Geometry: final body of the model. Coordinates: model frame, mm. Give positions to 0.01 mm unless a question says otherwise; leave off trailing zeros. Write each loop counter-clockwise with the first axis right and the second up, starting at its lowest first coordinate (ties: lowest second). Pieces come first, ordered by that corner, then holes.
from build123d import *

# Parameters (mm, degrees)
SKETCH1_W          = 520
SKETCH1_H          = 430
BASE_FLANGE1_DEPTH = 4.78
SKETCH6_R          = 4.5
CUT_EXTRUDE1_DEPTH = 10
CHAMFER1_SIZE      = 80
SKETCH7_R          = 4.5
CUT_EXTRUDE2_DEPTH = 10
SKETCH8_R          = 4.25
CUT_EXTRUDE3_DEPTH = 10
SKETCH9_R          = 4.5
CUT_EXTRUDE4_DEPTH = 10
CUT_EXTRUDE5_DEPTH = 10
CHAMFER2_SIZE      = 3


# Sheet-metal steps are written as plain solids
with BuildPart() as part:
    # Sketch1 → Base-Flange1 (new body)
    with BuildSketch(Plane(origin=(0, 0, 0), x_dir=(1, 0, 0), z_dir=(0, 1, 0))):
        with Locations((0, -215)):
            Rectangle(SKETCH1_W, SKETCH1_H)
    extrude(amount=-BASE_FLANGE1_DEPTH)

    # Sketch6 → Cut-Extrude1 (cut)
    with BuildSketch(Plane(origin=(0, 0, 0), x_dir=(1, 0, 0), z_dir=(0, 1, 0))):
        with Locations(Location((62.5, -14.9625, 0), (0, 0, 270))):
            Circle(SKETCH6_R)
        with Locations(Location((0, -14.9625, 0), (0, 0, 270))):
            Circle(SKETCH6_R)
        with Locations(Location((-62.5, -14.9625, 0), (0, 0, 270))):
            Circle(SKETCH6_R)
    extrude(amount=-CUT_EXTRUDE1_DEPTH, mode=Mode.SUBTRACT)

    # Chamfer1
    chamfer1_edges = [part.edges().sort_by_distance(p)[0] for p in [
        (260, -2.39, 430),
        (-260, -2.39, 430),
    ]]
    chamfer(chamfer1_edges, length=CHAMFER1_SIZE)

    # Sketch7 → Cut-Extrude2 (cut)
    with BuildSketch(Plane(origin=(0, 0, 0), x_dir=(1, 0, 0), z_dir=(0, 1, 0))):
        with Locations(Location((-223.749160028, -139.138800169, 0), (0, 0, 270))):
            Circle(SKETCH7_R)
        with Locations(Location((-223.749160028, -274.331266718, 0), (0, 0, 270))):
            Circle(SKETCH7_R)
        with Locations(Location((223.749160028, -274.331266718, 0), (0, 0, 90))):
            Circle(SKETCH7_R)
        with Locations(Location((223.749160028, -139.138800169, 0), (0, 0, 90))):
            Circle(SKETCH7_R)
    extrude(amount=-CUT_EXTRUDE2_DEPTH, mode=Mode.SUBTRACT)

    # Sketch8 → Cut-Extrude3 (cut)
    with BuildSketch(Plane(origin=(0, 0, 0), x_dir=(1, 0, 0), z_dir=(0, 1, 0))):
        with Locations(Location((46.669047558, -193.293452442, 0), (0, 0, 270))):
            Circle(SKETCH8_R)
        with Locations(Location((46.669047558, -286.631547558, 0), (0, 0, 270))):
            Circle(SKETCH8_R)
        with Locations(Location((-46.669047558, -286.631547558, 0), (0, 0, 270))):
            Circle(SKETCH8_R)
        with Locations(Location((-46.669047558, -193.293452442, 0), (0, 0, 270))):
            Circle(SKETCH8_R)
    extrude(amount=-CUT_EXTRUDE3_DEPTH, mode=Mode.SUBTRACT)

    # Sketch9 → Cut-Extrude4 (cut)
    with BuildSketch(Plane(origin=(0, 0, 0), x_dir=(1, 0, 0), z_dir=(0, 1, 0))):
        with Locations(Location((86.613706173, -164.085928216, 0), (0, 0, 270))):
            Circle(SKETCH9_R)
        with Locations(Location((86.613706173, -235.839071784, 0), (0, 0, 270))):
            Circle(SKETCH9_R)
        with Locations(Location((35.876571784, -113.348793827, 0), (0, 0, 270))):
            Circle(SKETCH9_R)
        with Locations(Location((-35.876571784, -113.348793827, 0), (0, 0, 270))):
            Circle(SKETCH9_R)
        with Locations(Location((-86.613706173, -164.085928216, 0), (0, 0, 270))):
            Circle(SKETCH9_R)
        with Locations(Location((-86.613706173, -235.839071784, 0), (0, 0, 270))):
            Circle(SKETCH9_R)
        with Locations(Location((0, -293.7125, 0), (0, 0, 270))):
            Circle(SKETCH9_R)
    extrude(amount=-CUT_EXTRUDE4_DEPTH, mode=Mode.SUBTRACT)

    # Sketch10 → Cut-Extrude5 (cut)
    with BuildSketch(Plane(origin=(0, 0, 0), x_dir=(1, 0, 0), z_dir=(0, 1, 0))):
        with BuildLine():
            Line((-14, -412.5), (-14, -387.5))
            ThreePointArc((-14, -387.5), (-10, -383.5), (-6, -387.5))
            Line((-6, -387.5), (-6, -412.5))
            ThreePointArc((-6, -412.5), (-10, -416.5), (-14, -412.5))
        make_face()
        with BuildLine():
            Line((-34, -412.5), (-34, -387.5))
            ThreePointArc((-34, -387.5), (-30, -383.5), (-26, -387.5))
            Line((-26, -387.5), (-26, -412.5))
            ThreePointArc((-26, -412.5), (-30, -416.5), (-34, -412.5))
        make_face()
        with BuildLine():
            Line((-54, -412.5), (-54, -387.5))
            ThreePointArc((-54, -387.5), (-50, -383.5), (-46, -387.5))
            Line((-46, -387.5), (-46, -412.5))
            ThreePointArc((-46, -412.5), (-50, -416.5), (-54, -412.5))
        make_face()
        with BuildLine():
            Line((-74, -412.5), (-74, -387.5))
            ThreePointArc((-74, -387.5), (-70, -383.5), (-66, -387.5))
            Line((-66, -387.5), (-66, -412.5))
            ThreePointArc((-66, -412.5), (-70, -416.5), (-74, -412.5))
        make_face()
        with BuildLine():
            Line((-94, -412.5), (-94, -387.5))
            ThreePointArc((-94, -387.5), (-90, -383.5), (-86, -387.5))
            Line((-86, -387.5), (-86, -412.5))
            ThreePointArc((-86, -412.5), (-90, -416.5), (-94, -412.5))
        make_face()
        with BuildLine():
            Line((14, -412.5), (14, -387.5))
            ThreePointArc((14, -387.5), (10, -383.5), (6, -387.5))
            Line((6, -387.5), (6, -412.5))
            ThreePointArc((6, -412.5), (10, -416.5), (14, -412.5))
        make_face()
        with BuildLine():
            Line((34, -412.5), (34, -387.5))
            ThreePointArc((34, -387.5), (30, -383.5), (26, -387.5))
            Line((26, -387.5), (26, -412.5))
            ThreePointArc((26, -412.5), (30, -416.5), (34, -412.5))
        make_face()
        with BuildLine():
            Line((54, -412.5), (54, -387.5))
            ThreePointArc((54, -387.5), (50, -383.5), (46, -387.5))
            Line((46, -387.5), (46, -412.5))
            ThreePointArc((46, -412.5), (50, -416.5), (54, -412.5))
        make_face()
        with BuildLine():
            Line((74, -412.5), (74, -387.5))
            ThreePointArc((74, -387.5), (70, -383.5), (66, -387.5))
            Line((66, -387.5), (66, -412.5))
            ThreePointArc((66, -412.5), (70, -416.5), (74, -412.5))
        make_face()
        with BuildLine():
            Line((94, -412.5), (94, -387.5))
            ThreePointArc((94, -387.5), (90, -383.5), (86, -387.5))
            Line((86, -387.5), (86, -412.5))
            ThreePointArc((86, -412.5), (90, -416.5), (94, -412.5))
        make_face()
    extrude(amount=-CUT_EXTRUDE5_DEPTH, mode=Mode.SUBTRACT)

    # Chamfer2
    chamfer2_edges = [part.edges().sort_by_distance(p)[0] for p in [
        (62.5, 0, 10.4625),
        (0, 0, 10.4625),
        (-62.5, 0, 10.4625),
        (-223.749160028, 0, 134.638800169),
        (-223.749160028, 0, 269.831266718),
        (223.749160028, 0, 278.831266718),
        (223.749160028, 0, 143.638800169),
    ]]
    chamfer(chamfer2_edges, length=CHAMFER2_SIZE)


solid = part.part
Q1. Section B-B on x = 202. Output: boundary loops of the cut face in (y, z), plus the area to 3 significant figures.
Filled sheet:
outline: (-4.78, 0) - (0, 0) - (0, 408) - (-4.78, 408) - close
area: 1,950 mm2
Q2. Pin query (flat end, axial travel): P1, Ø1, axis at x = -87.5, z = 325, coming from the +Y side; P2, Ø2.5, axis at y = -3, z = 405.5, coming from the +X side; P3, Ø1.4, axis at y = -1.5, z = 396, coming from the -X side; P4, Ø1.4, axis at y = -2, z = 397.5, coming from the +X side. Return the tip coordinate at first contact, or that it passes through.
Filled sheet:
P1: stops at y = 0
P2: stops at x = 205.75
P3: stops at x = -214.7
P4: stops at x = 213.2
Q3. Pull-direction query (Z, two-part tool) for faces 1 (the flat face through (221, -2, 389)), 2 (the flat face through (-4, -4.78, 212)), 3 (the conical face through (67.11, -2.85, 14.36)), 4 (the conical face through (-228.284, -2.854, 138.132)); classes: released by +Z, released by -Z, zero draft, split by the parting line, or undercut.
Filled sheet:
face 1: released by +Z
face 2: zero draft
face 3: undercut
face 4: undercut
Q4. Section A-A on z = 394. Count the separate pieces of the cut face and the enclosed holes in it, plus the area to 3 significant figures.
Filled sheet:
separate pieces: 11
enclosed holes: 0
area: 1,680 mm2
Q5. Ray query, line 1 along X through (y, z) = (-2.95, 274.5); line 2 along X through (y, z) = (-0.4, 293); line 3 along X through (y, z) = (-2.85, 277). Return the intervals inside material, ascending.
Filled sheet:
line 1: x = -260 to -228.3, -219.2 to 219.2, 228.3 to 260
line 2: x = -260 to -4.44, 4.44 to 260
line 3: x = -260 to -227.56, -219.94 to 219.94, 227.56 to 260
